from build123d import *

# Parameters (mm, degrees)
F0_W     = 508
F0_H     = 50.8
F1_DEPTH = 12.7
F3_D     = 6.5278
F5_D     = 13.49248


with BuildPart() as f1:
    # F0 (on Front) → F1 (new body)
    with BuildSketch(Plane.XZ):
        Rectangle(F0_W, F0_H)
    extrude(amount=F1_DEPTH)

    # F3 (through all)
    with Locations(Plane.XZ.offset(12.7)):
        with Locations((-203.2, 19.05), (203.2, 19.05), (-203.2, -19.05), (203.2, -19.05)):
            Hole(F3_D / 2)

    # F5 (through all)
    with Locations(Plane.XZ.offset(12.7)):
        with Locations((165.1, 0), (-165.1, 0)):
            Hole(F5_D / 2)


solid = f1.part
Here's how the part is built. I have some questions about the finished solid (model axes, mm). Round coordinates to 2 decimals unless told otherwise and drop trailing zeros. Order: outer loops, then holes, each group sorted by start corner. A loop starts at its lowest first (then second) coordinate and runs counter-clockwise, first axis right, second up. Notation, with made-up numbers: (-20, 44.25) -> (-5, 44.25) arc R29 cw to (-5, 74.25) -> close; hole circle Ø4 at (53.25, -19.75). An arc over 180 degrees is marked (long way). Return JSON: item names as keys, results as strings.
Q1. I need wall thicknesses on line 1 along Z through (x, y) = (-203.2, -6.25); line 2 along X through (y, z) = (-4, 19); line 3 along X through (y, z) = (-1.5, -0.5). Which ranges of each line are inside material? Lowest first, please. Write a range as from..to.
Filled sheet:
{"line 1": "z = -25.4..-22.31, -15.79..15.79, 22.31..25.4", "line 2": "x = -254..-206.46, -199.94..199.94, 206.46..254", "line 3": "x = -254..-171.83, -158.37..158.37, 171.83..254"}
Q2. If we section it at B-B on y = -4.25: List the corners of the cut face in (x, z) for me.
Filled sheet:
{"outline": "(-254, -25.4) -> (254, -25.4) -> (254, 25.4) -> (-254, 25.4) -> close; hole circle Ø6.53 at (-203.2, -19.05); hole circle Ø6.53 at (-203.2, 19.05); hole circle Ø13.49 at (-165.1, 0); hole circle Ø13.49 at (165.1, 0); hole circle Ø6.53 at (203.2, -19.05); hole circle Ø6.53 at (203.2, 19.05)"}
Q3. If we section it at A-A on x = 165.1: List the corners of the cut face in (y, z) for me, plus the area to 3 significant figures.
Filled sheet:
{"outline": "(-12.7, -25.4) -> (0, -25.4) -> (0, -6.75) -> (-12.7, -6.75) -> close; (-12.7, 6.75) -> (0, 6.75) -> (0, 25.4) -> (-12.7, 25.4) -> close", "area": "474 mm^2"}
Q4. If we mould it in two halves opening along Z, with no side actions, what happens to faces 1 (the flat face through (-4, -6, 25.4)), 2 (the cylindrical face through (171.84, -6.26, 0.3)), 3 (the flat face through (-4, -12.7, 0))? For each: released by +Z, released by -Z, zero draft, split by the parting line, or undercut.
Filled sheet:
{"face 1": "released by +Z", "face 2": "undercut", "face 3": "zero draft"}
